from build123d import *

# Parameters (mm, degrees)
PAD_DEPTH = 35
FILLET_R  = 1.4


with BuildPart() as part:
    # Sketch → Pad (new body)
    with BuildSketch(Plane.XY):
        Polygon((-9, 0), (9, 0), (9, 3), (1.5, 3), (1.5, 23), (-1.5, 23), (-1.5, 3), (-9, 3), align=None)
    extrude(amount=PAD_DEPTH)

    # Fillet
    fillet_edges = [part.edges().sort_by_distance(p)[0] for p in [
        (9, 3, 17.5),
        (-9, 3, 17.5),
        (1.5, 3, 17.5),
        (-1.5, 3, 17.5),
        (1.5, 23, 17.5),
        (-1.5, 23, 17.5),
    ]]
    fillet(fillet_edges, radius=FILLET_R)


solid = part.part
The model under review builds one solid part; all positions refer to its coordinate system, in mm. A direction names the side the tool comes from. Round coordinates to 2 decimals unless told otherwise and drop trailing zeros. Loops run counter-clockwise (first coordinate to the right, second up) from the corner with the lowest first, then second, coordinate; pieces in that order, holes last. Notation, with made-up numbers: (-27, 25.25) -> (20, 25.25) arc R17 ccw to (20, 41.25) -> close; hole circle Ø10 at (-18, 85.25). An arc over 180 degrees is marked (long way). Answer as CSV lines item,"result".
1) Add section A-A on z = 4. Write out the cut boundary in (x, y).
Geometry results:
outline,"(-9, 0) -> (9, 0) -> (9, 1.6) arc R1.4 ccw to (7.6, 3) -> (2.9, 3) arc R1.4 cw to (1.5, 4.4) -> (1.5, 21.6) arc R1.4 ccw to (0.1, 23) -> (-0.1, 23) arc R1.4 ccw to (-1.5, 21.6) -> (-1.5, 4.4) arc R1.4 cw to (-2.9, 3) -> (-7.6, 3) arc R1.4 ccw to (-9, 1.6) -> close"
2) Add section B-B on x = 6.25. Write out the cut boundary in (y, z), plus the area to 3 significant figures.
Geometry results:
outline,"(0, 0) -> (3, 0) -> (3, 35) -> (0, 35) -> close"
area,"105 mm²"
3) Add section C-C on y = 13.5. Write out the cut boundary in (x, z).
Geometry results:
outline,"(-1.5, 0) -> (1.5, 0) -> (1.5, 35) -> (-1.5, 35) -> close"
4) To check wall thickness, follow line 1 along X through (y, z) = (19.75, 6); line 2 along Y through (x, z) = (6.5, 32); line 3 along Y through (x, z) = (1.25, 11). State the ranges of each line that lie inside material, in increasing order. Write a range as from..to.
Geometry results:
line 1,"x = -1.5..1.5"
line 2,"y = 0..3"
line 3,"y = 0..22.4"
5) Tool access review of faces 1 (the face through (-5, 3, 17)), 2 (the face through (0, 0, 17)), 3 (the face through (1.5, 13, 17)): name each direction out of +Z, -Z, +X, -X, +Y, -Y from which nothing blocks a thin tool from reaching the whole face with its end or side.
Geometry results:
face 1,"+Z, -Z, -X, +Y"
face 2,"+Z, -Z, +X, -X, -Y"
face 3,"+Z, -Z, +X, +Y"
6) For P1, Ø2, axis at y = 10.5, z = 18.5, coming from the +X side; P2, Ø1.4, axis at x = -6, z = 13, coming from the +Y side; P3, Ø4, axis at y = 11.5, z = 13, coming from the -X side, all flat-tipped, find the tip position at first contact; note any pin that passes through.
Geometry results:
P1,"stops at x = 1.5"
P2,"stops at y = 3"
P3,"stops at x = -1.5"
